For this review, take the finished solid that the model builds, in its own axes (mm). Face numbers are marked on the shaded views. A direction names the side the tool comes from. Round coordinates to 2 decimals unless told otherwise and drop trailing zeros. Write each loop counter-clockwise with the first axis right and the second up, starting at its lowest first coordinate (ties: lowest second). Pieces come first, ordered by that corner, then holes. Notation, with made-up numbers: (87.5, -34) - (106.5, -34) arc R19 cw to (106.5, 2) - close; hole circle Ø11 at (34, 38). An arc over 180 degrees is marked (long way). One line per item, written item: value. Start each with the question number.
Q1. Add section C-C on z = -4.25. Write out the cut boundary in (x, y), and give its area (3 significant figures).
Q2. Add section D-D on y = -10. Write out the cut boundary in (x, z).
Q3. Add section A-A on x = 0. Write out the cut boundary in (y, z).
Q4. Tool access review of the marked faces 5, 6, 7, 8 and 9: name each direction out of +Z, -Z, +X, -X, +Y, -Y from which nothing blocks a thin tool from reaching the whole face with its end or side.
Q5. Mouldability with a two-part tool opening along X and no side actions: class the marked faces 1, 2, 3 and 4 as +X half, -X half, draft (parallel to the pull), parting line (faces both ways), or undercut.
Q6. Add section B-B on z = 9.75. Write out the cut boundary in (x, y).
Q7. For probe 1 along Z at (x, y) = (0, 1.45); probe 2 along X at (y, z) = (1.4, 9); probe 3 along Z at (x, y) = (11.75, -16.75), list the stretches that pass through material, from the lowest coordinate up.
Q8. Clearance check with flat-ended pins moving along their axes: pin 1 Ø10 at (x, y) = (8.5, -11) entering from -Z; pin 2 Ø8 at (x, z) = (-1.5, -6) entering from -Y; pin 3 Ø9.5 at (y, z) = (-8, 2) entering from -X. State where each tip first meets the part, or that it passes through.
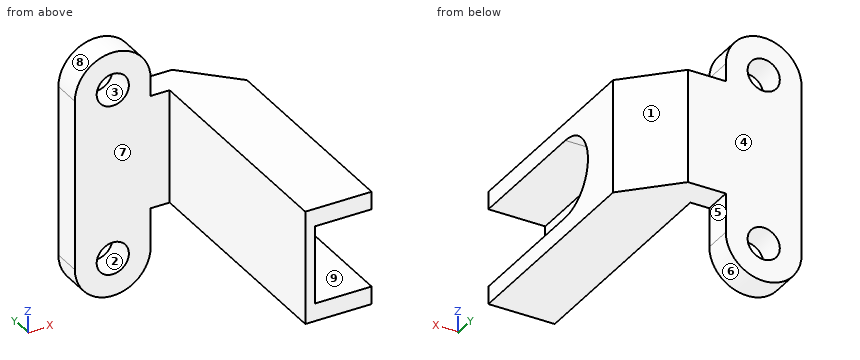
```python
from build123d import *

# Parameters (mm, degrees)
BOSS_EXTRUDE1_DEPTH      = 3
M3_CLEARANCE_HOLE1_D     = 3.4
M3_CLEARANCE_HOLE1_DEPTH = 10
M3_CLEARANCE_HOLE1_TIP   = 1.021463052
SKETCH2_W                = 7
SKETCH2_H                = 12
BOSS_EXTRUDE2_DEPTH      = 24.7
CUT_EXTRUDE1_DEPTH       = 6
CHAMFER3_SIZE            = 5


with BuildPart() as part:
    # Sketch1 → Boss-Extrude1 (new body)
    with BuildSketch(Plane(origin=(0, 0, 0), x_dir=(1, 0, 0), z_dir=(0, 1, 0))):
        with BuildLine():
            ThreePointArc((-4, -9), (0, -13), (4, -9))
            Line((4, -9), (4, -7.132441433))
            Line((4, -7.132441433), (13, -7.132441433))
            Line((13, -7.132441433), (13, 4.867558567))
            Line((13, 4.867558567), (4, 4.867558567))
            Line((4, 4.867558567), (4, 9))
            ThreePointArc((4, 9), (0, 13), (-4, 9))
            Line((-4, 9), (-4, 4.867558567))
            Line((-4, 4.867558567), (-4, -9))
        make_face()
    extrude(amount=BOSS_EXTRUDE1_DEPTH)

    # M3 Clearance Hole1
    with Locations(Plane(origin=(0, 3, 0), x_dir=(1, 0, 0), z_dir=(0, 1, 0))):
        with Locations((0, -9), (0, 9)):
            Hole(M3_CLEARANCE_HOLE1_D / 2, depth=M3_CLEARANCE_HOLE1_DEPTH)
            with Locations((0, 0, -(M3_CLEARANCE_HOLE1_DEPTH + M3_CLEARANCE_HOLE1_TIP / 2))):  # 118° drill point
                Cone(0, M3_CLEARANCE_HOLE1_D / 2, M3_CLEARANCE_HOLE1_TIP, mode=Mode.SUBTRACT)

    # Sketch2 → Boss-Extrude2 (add)
    with BuildSketch(Plane.XZ):
        with Locations((9.5, 1.132441433)):
            Rectangle(SKETCH2_W, SKETCH2_H)
    extrude(amount=BOSS_EXTRUDE2_DEPTH)

    # Sketch3 → Cut-Extrude1 (cut)
    with BuildSketch(Plane(origin=(13, 0, 0), x_dir=(0, 0, -1), z_dir=(1, 0, 0))):
        with BuildLine():
            Line((2.992558567, -24.7), (-5.257441433, -24.7))
            Line((-5.257441433, -24.7), (-5.257441433, -10.7))
            ThreePointArc((-5.257441433, -10.7), (-1.132441433, -6.575), (2.992558567, -10.7))
            Line((2.992558567, -10.7), (2.992558567, -24.7))
        make_face()
    extrude(amount=-CUT_EXTRUDE1_DEPTH, mode=Mode.SUBTRACT)

    # Chamfer3
    chamfer3_edges = [part.edges().sort_by_distance(p)[0] for p in [
        (13, 3, 1.132441433),
    ]]
    chamfer(chamfer3_edges, length=CHAMFER3_SIZE)


solid = part.part
```
Result set:
1. outline: (-4, 0) - (6, 0) - (6, -24.7) - (13, -24.7) - (13, -2) - (8, 3) - (-4, 3) - close
1. area: 211 mm^2
2. outline: (6, -4.87) - (13, -4.87) - (13, -2.93) - (7, -2.93) - (7, 5.2) - (13, 5.2) - (13, 7.13) - (6, 7.13) - close
3. outline: (0, -13) - (3, -13) - (3, -10.7) - (0, -10.7) - close; (0, -7.3) - (3, -7.3) - (3, 7.3) - (0, 7.3) - close; (0, 10.7) - (3, 10.7) - (3, 13) - (0, 13) - close
4. face 5: -Z, +X, +Y, -Y
4. face 6: -Z, +Y, -Y
4. face 7: +Z, -Z, -X, -Y
4. face 8: +Z, +Y, -Y
4. face 9: +X, -Y
5. face 1: +X half
5. face 2: undercut
5. face 3: undercut
5. face 4: draft
6. outline: (-3.93, 0) - (-1.53, 0) - (-1.53, 3) - (-3.93, 3) - close; (1.53, 0) - (3.93, 0) - (3.93, 3) - (1.53, 3) - close
7. probe 1: z = -13 to -10.7, -7.3 to 7.3, 10.7 to 13
7. probe 2: x = -4 to -1.7, 1.7 to 4
7. probe 3: z = -4.87 to -2.99, 5.26 to 7.13
8. pin 1: stops at z = -4.87
8. pin 2: stops at y = 0
8. pin 3: stops at x = 6
